Source: CAD feature listing. Evaluate the final solid. Frame: model axes, mm. Give positions to 0.01 mm unless a question says otherwise; leave off trailing zeros. Loops run counter-clockwise (first coordinate to the right, second up) from the corner with the lowest first, then second, coordinate; pieces in that order, holes last.
from build123d import *
from build123d.topology import SkipClean

# Parameters (mm, degrees)
SHAFT_DEPTH                     = 130
SHAFT_DEPTH_BACK                = 130
SKETCH2_R                       = 5
SHAFT_KEY_FOR_BICEPS_DEPTH      = 130
SHAFT_KEY_FOR_BICEPS_DEPTH_BACK = 30
SKETCH3_W                       = 5
SKETCH3_H                       = 8
CUT_EXTRUDE1_START              = -75
CUT_EXTRUDE1_DEPTH              = 75
CUT_EXTRUDE2_START              = -25
CUT_EXTRUDE2_DEPTH              = 25
BOSS_EXTRUDE1_DEPTH             = 15


with BuildPart() as part:
    # Sketch2 → Shaft (new, two sides: drawn at the far end of the back side and taken through both)
    with BuildSketch(Plane(origin=(0, 0, 0), x_dir=(0, 0, -1), z_dir=(1, 0, 0)).offset(-SHAFT_DEPTH_BACK)):
        Circle(SKETCH2_R)
    extrude(amount=SHAFT_DEPTH + SHAFT_DEPTH_BACK)

    # Sketch3 → Shaft Key for Biceps (add, two sides: drawn at the far end of the back side and taken through both)
    with BuildSketch(Plane(origin=(0, 0, 0), x_dir=(0, 0, -1), z_dir=(1, 0, 0)).offset(-SHAFT_KEY_FOR_BICEPS_DEPTH_BACK)):
        with Locations((0, 4)):
            Rectangle(SKETCH3_W, SKETCH3_H)
    extrude(amount=SHAFT_KEY_FOR_BICEPS_DEPTH + SHAFT_KEY_FOR_BICEPS_DEPTH_BACK)

    # Sketch5 → Cut-Extrude1 (cut)
    with BuildSketch(Plane(origin=(130, 0, 0), x_dir=(0, 0, -1), z_dir=(1, 0, 0)).offset(CUT_EXTRUDE1_START)):
        with BuildLine():
            Line((-2.5, 4.330127019), (-2.5, 8))
            Line((-2.5, 8), (2.5, 8))
            Line((2.5, 8), (2.5, 4.330127019))
            ThreePointArc((2.5, 4.330127019), (0, 5), (-2.5, 4.330127019))
        make_face()
    extrude(amount=CUT_EXTRUDE1_DEPTH, mode=Mode.SUBTRACT)

    # Sketch9 → Cut-Extrude2 (cut)
    with SkipClean():  # the faces are left unmerged after this step: merging them gives an invalid solid
        with BuildSketch(Plane(origin=(55, 0, 0), x_dir=(0, 0, -1), z_dir=(1, 0, 0)).offset(CUT_EXTRUDE2_START)):
            with BuildLine():
                Line((2.5, 4.330127019), (2.5, 8))
                Line((2.5, 8), (-2.5, 8))
                Line((-2.5, 8), (-2.5, 4.330127019))
                ThreePointArc((-2.5, 4.330127019), (0, 5), (2.5, 4.330127019))
            make_face()
        extrude(amount=CUT_EXTRUDE2_DEPTH, mode=Mode.SUBTRACT)

    # Sketch10 → Boss-Extrude1 (add)
    with SkipClean():  # the faces are left unmerged after this step: merging them gives an invalid solid
        with BuildSketch(Plane(origin=(55, 0, 0), x_dir=(0, 0, -1), z_dir=(1, 0, 0))):
            with BuildLine():
                Line((-2.5, 8), (-2.5, 4.330127019))
                ThreePointArc((-2.5, 4.330127019), (0, 5), (2.5, 4.330127019))
                Line((2.5, 4.330127019), (2.5, 8))
                Line((2.5, 8), (-2.5, 8))
            make_face()
        extrude(amount=BOSS_EXTRUDE1_DEPTH)


solid = part.part
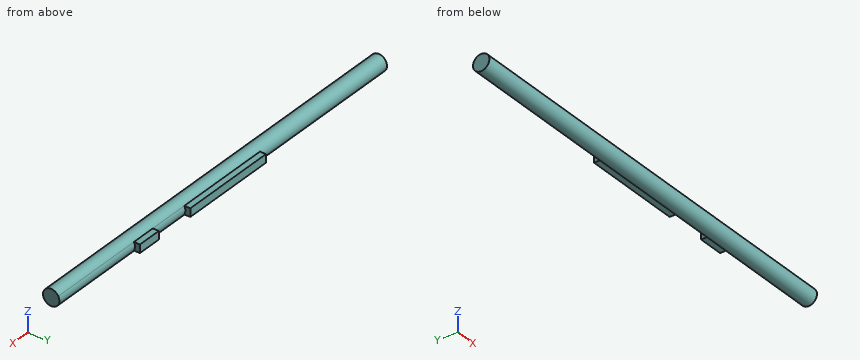
1) Cut plane D-D (x = 63). Return loops of the section in (y, z), and give its area (3 significant figures).
Checks:
outline: (4.33, -2.5) - (8, -2.5) - (8, 2.5) - (4.33, 2.5) arc R5 ccw (long way) to start
area: 94.6 mm2
2) Cut plane B-B (x = -61). Return loops of the section in (y, z), and give its area (3 significant figures).
Checks:
outline: circle Ø10 at (0, 0)
area: 78.5 mm2
3) Cut plane C-C (y = 2.25). Return loops of the section in (x, z).
Checks:
outline: (-130, -4.47) - (130, -4.47) - (130, 4.47) - (-130, 4.47) - close
4) Contact query for flat-ended pins moving along their axis: P1, Ø1.1, axis at x = 65.5, y = 7, coming from the +Z side; P2, Ø1.8, axis at y = 6, z = 0.5, coming from the -X side; P3, Ø4, axis at x = -13.5, y = 5.5, coming from the -Z side. Output: stop coordinate, or through.
Checks:
P1: stops at z = 2.5
P2: stops at x = -30
P3: stops at z = -3.57
5) Cut plane A-A (z = 0). Return loops of the section in (x, y), and give its area (4 significant figures).
Checks:
outline: (-130, -5) - (130, -5) - (130, 5) - (70, 5) - (70, 8) - (55, 8) - (55, 5) - (30, 5) - (30, 8) - (-30, 8) - (-30, 5) - (-130, 5) - close
area: 2,825 mm2
6) Ray query, probe 1 along X at (y, z) = (6.5, -2.25); probe 2 along Y at (x, z) = (17.5, 0.5); probe 3 along Z at (x, y) = (24.5, 6.75). Return the intervals inside material, ascending.
Checks:
probe 1: x = -30 to 30, 55 to 70
probe 2: y = -4.97 to 8
probe 3: z = -2.5 to 2.5
